Check sheet for the modelled part. Datum: model origin and axes. Units: mm. A direction names the side the tool comes from. Give positions to 0.01 mm unless a question says otherwise; leave off trailing zeros. Write each loop counter-clockwise with the first axis right and the second up, starting at its lowest first coordinate (ties: lowest second). Pieces come first, ordered by that corner, then holes. Notation, with made-up numbers: M 80,47 L 113,47 A27 ccw 113,83 Z; hole C -27,3.25 d11. An arc over 180 degrees is marked long. Write item = value, one per line. Start each with the question number.
1) Gauge pin test, flat ends, axial feed: pin 1 (2 mm diameter, centred on x = 25.5, z = 37, fed in from -Y); pin 2 (6 mm diameter, centred on y = 10, z = 53, fed in from +X); pin 3 (8 mm diameter, centred on x = 48, z = 27, fed in from +Y); pin 4 (8.5 mm diameter, centred on y = -15.5, z = 17, fed in from -X) (3 decimals). Record the tip position at first contact, or that the pin passes through.
2) Set-up check for faces 1 (the face through (30.78, -16.79, 49.9)), 2 (the face through (60, -2, 61.925)), 3 (the face through (41.275, -1, 4)), 4 (the face through (60, 2, 42.875)), 5 (the face through (-5, 7.938, 30)): record each of +Z, -Z, +X, -X, +Y, -Y from which the full face is reachable in a straight line by a thin tool's end or side.
3) Scan lines: L1, parallel to X at y = -34.5, z = 6 (3 decimals); L2, parallel to X at y = 24, z = 21 (3 decimals); L3, parallel to Y at x = 49, z = 42.5. Record each from-to range of solid material in increasing order.
4) Sectioned sample at B-B, the plane x = 91. Record the cut outline in (y, z) (3 decimals), then the cut area to 3 significant figures.
5) Sectioned sample at A-A, the plane y = -44. Record the cut outline in (x, z) (3 decimals).
from build123d import *

# Parameters (mm, degrees)
F1_DEPTH = 63.5
F2_DEPTH = 7.9375
F0_W     = 25.4
F0_H     = 19.05
F3_DEPTH = 25.4
F5_R     = 6.35


with BuildPart() as f1:
    # F0 (on Front) → F1 (new body, symmetric)
    with BuildSketch(Plane.XZ):
        Polygon((-41.275, -9.525), (41.275, -9.525), (41.275, 9.525), (22.225, 9.525), (-41.275, 9.525), align=None)
    extrude(amount=F1_DEPTH, both=True)

    # F0 (on Front) → F2 (join, symmetric)
    with BuildSketch(Plane.XZ):
        with BuildLine():
            add(Edge.make_bspline(
                [(-41.275, 9.525), (-41.6549469466, 29.246440989), (16.2084851721, 57.3919038747), (51.5697219999, 61.4765124832)],
                knots=[0, 0, 0, 0, 105.7290350632, 105.7290350632, 105.7290350632, 105.7290350632], degree=3))
            Line((-41.275, 9.525), (22.225, 9.525))
            Line((22.225, 9.525), (22.225, 27.0002))
            ThreePointArc((22.225, 27.0002), (30.5544474192, 49.6371655193), (51.5697219999, 61.4765124832))
        make_face()
    extrude(amount=F2_DEPTH, both=True)

    # F0 (on Front) → F3 (join, symmetric)
    with BuildSketch(Plane.XZ):
        with BuildLine():
            Line((22.225, 9.525), (41.275, 9.525))
            Line((41.275, 9.525), (41.275, 27.0002))
            ThreePointArc((41.275, 27.0002), (45.9246798487, 38.2255201513), (57.15, 42.8752))
            Line((57.15, 42.8752), (60.325, 42.8752))
            Line((60.325, 42.8752), (60.325, 61.9252))
            Line((60.325, 61.9252), (57.15, 61.9252))
            add(Edge.make_bspline(
                [(51.5697219999, 61.4765124832), (53.5013471404, 61.699636259), (55.3658269691, 61.8509637705), (57.15, 61.9252)],
                knots=[105.7290350632, 105.7290350632, 105.7290350632, 105.7290350632, 111.5045361635, 111.5045361635, 111.5045361635, 111.5045361635], degree=3))
            ThreePointArc((51.5697219999, 61.4765124832), (30.5544474192, 49.6371655193), (22.225, 27.0002))
            Line((22.225, 27.0002), (22.225, 9.525))
        make_face()
        with Locations((73.025, 52.4002)):
            Rectangle(F0_W, F0_H)
    extrude(amount=F3_DEPTH, both=True)

    # F0 (on Front) → F4 (revolve)
    with BuildSketch(Plane.XZ):
        Polygon((85.725, 61.9252), (85.725, 42.8752), (85.725, 38.1), (111.125, 38.1), (111.125, 66.675), (85.725, 66.675), align=None)
    revolve(axis=Axis((85.725, 0, 52.3875), (0, 0, 1)))

    # F5
    f5_edges = [f1.edges().sort_by_distance(p)[0] for p in [
        (41.275, -63.5, 0),
        (-41.275, -63.5, 0),
        (-41.275, 63.5, 0),
        (41.275, 63.5, 0),
    ]]
    fillet(f5_edges, radius=F5_R)


solid = f1.part
Data:
q1.pin_1 = -25.4
q1.pin_2 = 110.14
q1.pin_3 = through
q1.pin_4 = 22.225
q2.face_1 = +Z, -X, -Y
q2.face_2 = +Z, -X
q2.face_3 = -Z, +X, +Y, -Y
q2.face_4 = -Z
q2.face_5 = +Z, -X, +Y
q3.L1 = -41.275 to 41.275
q3.L2 = 22.225 to 41.275
q3.L3 = -25.4 to 25.4
q4.outline = M -24.846,38.1 L 24.846,38.1 L 24.846,66.675 L -24.846,66.675 Z
q4.area = 1,420 mm2
q5.outline = M -41.275,-9.525 L 41.275,-9.525 L 41.275,9.525 L -41.275,9.525 Z
